Here's how the part is built. I have some questions about the finished solid (model axes, mm). Coordinates: 2 decimals unless noted, no trailing zeros. Loops run counter-clockwise (first coordinate to the right, second up) from the corner with the lowest first, then second, coordinate; pieces in that order, holes last. Notation, with made-up numbers: (71, 18) -> (109, 18) arc R23 ccw to (109, 45) -> close; hole circle Ø7 at (-1, -30). An arc over 180 degrees is marked (long way). Answer as a JSON object with one key per item and string values. Group by question number.
1) I need wall thicknesses on probe 1 along X at (y, z) = (-25.5, 17); probe 2 along Z at (x, y) = (-11, -0.8); probe 3 along Z at (x, y) = (7, -24). Which ranges of each line are inside material? Lowest first, please. Write a range as [from, to].
2) I want a section at A-A (z = 0). Write out the boundary of the cut face in (x, y).
3) I'm going to push flat-ended pins straight in: pin 1 (6 mm diameter, centred on y = -2.5, z = -14, fed in from -X); pin 2 (1.6 mm diameter, centred on x = -11, z = 31.24, fed in from +Y); pin 3 (6 mm diameter, centred on y = 28, z = -28.5, fed in from -X); pin 4 (9.5 mm diameter, centred on y = 0, z = 0, fed in from +X). Where does each tip first touch, or does it pass through?
4) I want a section at B-B (y = 0). Write out the boundary of the cut face in (x, z).
5) I want a section at C-C (x = -11). Write out the boundary of the cut face in (y, z).
6) I want a section at D-D (x = -5.25). Write out the boundary of the cut face in (y, z), then the cut area to 3 significant figures.
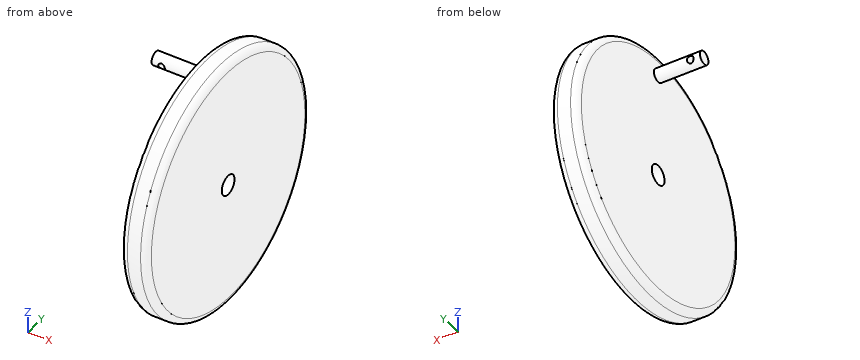
Autodesk Inventor part; units mm, degrees
ref_plane "YZ Plane" through (0, 0, 0) normal (1, 0, 0) x (0, 1, 0)
ref_plane "XZ Plane" through (0, 0, 0) normal (0, 1, 0) x (-1, 0, 0)
ref_plane "XY Plane" through (0, 0, 0) normal (0, 0, 1) x (1, 0, 0)
sketch "Sketch1" plane through (0, 0, 0) normal (1, 0, 0) x (0, 1, 0)
  circle A0 centre (0, 0) radius 38.1
  circle A1 centre (0, 31.6517) radius 2
  dimension "d0" = 76.2
  dimension "d14" = 4
extrude "Extrusion1" add sketch "Sketch1" along normal blind 8 contours A0 | A1
sketch "Sketch2" plane through (8, 0, 0) normal (1, 0, 0) x (0, 0, -1)
  circle A0 centre (0, 0) radius 3
  dimension "d3" = 6
extrude "Extrusion2" cut sketch "Sketch2" against normal through all
fillet "Fillet1" radius 2 2 edges at (8, -38.1, 0) (0, -38.1, 0)
sketch "Sketch4" plane through (8, 0, 0) normal (1, 0, 0) x (0, 0, -1)
  point P0 (0, 0)
sketch "Sketch7" plane through (8, 0, 0) normal (1, 0, 0) x (0, 0, -1)
  point P0 (0, 0)
extrude "Extrusion5" add sketch "Sketch1" against normal blind 14 contours A1
sketch "Sketch8" plane through (0, 0, 0) normal (0, 1, 0) x (-1, 0, 0)
  circle A0 centre (11, 31.2419) radius 1
  line L0 (14, 29.6517) -> (14, 33.6517)
  point P0 (0, 0)
  dimension "d17" = 2
  dimension "d18" = 3
extrude "Extrusion6" cut sketch "Sketch8" along normal mid plane 14
properties part number "extension circle" material "Brass, Soft Yellow"
Determined:
{
 "1": {"probe 1": "[0, 8]", "probe 2": "[29.82, 30.24], [32.24, 33.48]", "probe 3": "[-29.24, 29.24]"},
 "2": {"outline": "(0, -36.1) arc R2 ccw to (2, -38.1) -> (6, -38.1) arc R2 ccw to (8, -36.1) -> (8, -3) -> (0, -3) -> close; (0, 3) -> (8, 3) -> (8, 36.1) arc R2 ccw to (6, 38.1) -> (2, 38.1) arc R2 ccw to (0, 36.1) -> close"},
 "3": {"pin 1": "x = 0", "pin 2": "through", "pin 3": "x = 0.19", "pin 4": "x = 8"},
 "4": {"outline": "(-14, 29.65) -> (0, 29.65) -> (0, 3) -> (8, 3) -> (8, 36.1) arc R2 ccw to (6, 38.1) -> (2, 38.1) arc R2 ccw to (0, 36.1) -> (0, 33.65) -> (-14, 33.65) -> close; (0, -36.1) arc R2 ccw to (2, -38.1) -> (6, -38.1) arc R2 ccw to (8, -36.1) -> (8, -3) -> (0, -3) -> close; hole circle Ø2 at (-11, 31.24)"},
 "5": {"outline": "(-1.91, 32.24) -> (1.91, 32.24) arc R2 ccw to start; (-1.42, 30.24) arc R2 ccw to (1.42, 30.24) -> close"},
 "6": {"outline": "circle Ø4 at (0, 31.65)", "area": "12.6 mm^2"}
}
